Geometry check sheet. Reference: the model listing, model coordinates, mm. Face numbers are marked on the shaded views. A direction names the side the tool comes from. Coordinates: 2 decimals unless noted, no trailing zeros. Loops run counter-clockwise (first coordinate to the right, second up) from the corner with the lowest first, then second, coordinate; pieces in that order, holes last. Notation, with made-up numbers: M 57.5,83 L 110.5,83 A28 cw 110.5,115 Z; hole C 35.5,20.5 d4. An arc over 180 degrees is marked long. Use CSV: the item, a comma, the result in double quotes.
```python
from build123d import *

# Parameters (mm, degrees)
SKETCH1_W           = 16
SKETCH1_H           = 30
BOSS_EXTRUDE1_DEPTH = 9
SKETCH2_R           = 3
BOSS_EXTRUDE2_DEPTH = 1
SKETCH3_R           = 3
BOSS_EXTRUDE3_DEPTH = 2
BOSS_EXTRUDE4_DEPTH = 30
SKETCH6_R           = 0.75
BOSS_EXTRUDE5_DEPTH = 10
SKETCH7_R           = 3.5
BOSS_EXTRUDE6_DEPTH = 4


with BuildPart() as part:
    # Sketch1 → Boss-Extrude1 (new body, symmetric)
    with BuildSketch(Plane(origin=(0, 0, 0), x_dir=(1, 0, 0), z_dir=(0, 1, 0))):
        with Locations((0, -15)):
            Rectangle(SKETCH1_W, SKETCH1_H)
    extrude(amount=BOSS_EXTRUDE1_DEPTH, both=True)

    # Sketch2 → Boss-Extrude2 (add)
    with BuildSketch(Plane(origin=(0, 0, 0), x_dir=(-1, 0, 0), z_dir=(0, 0, -1))):
        Circle(SKETCH2_R)
    extrude(amount=BOSS_EXTRUDE2_DEPTH)

    # Sketch3 → Boss-Extrude3 (add)
    with BuildSketch(Plane.XY.offset(30)):
        Circle(SKETCH3_R)
    extrude(amount=BOSS_EXTRUDE3_DEPTH)

    # Sketch5 → Boss-Extrude4 (add)
    with BuildSketch(Plane.XY):
        with BuildLine():
            Line((8, 9), (8, -9))
            ThreePointArc((8, -9), (12, 0), (8, 9))
        make_face()
        with BuildLine():
            Line((-8, 9), (-8, -9))
            ThreePointArc((-8, -9), (-12, 0), (-8, 9))
        make_face()
    extrude(amount=BOSS_EXTRUDE4_DEPTH)

    # Sketch6 → Boss-Extrude5 (add)
    with BuildSketch(Plane(origin=(0, 0, 0), x_dir=(-1, 0, 0), z_dir=(0, 0, -1))):
        Circle(SKETCH6_R)
    extrude(amount=BOSS_EXTRUDE5_DEPTH)

    # Sketch7 → Boss-Extrude6 (add)
    with BuildSketch(Plane(origin=(0, 0, -10), x_dir=(-1, 0, 0), z_dir=(0, 0, -1))):
        Circle(SKETCH7_R)
    extrude(amount=-BOSS_EXTRUDE6_DEPTH)


solid = part.part
```
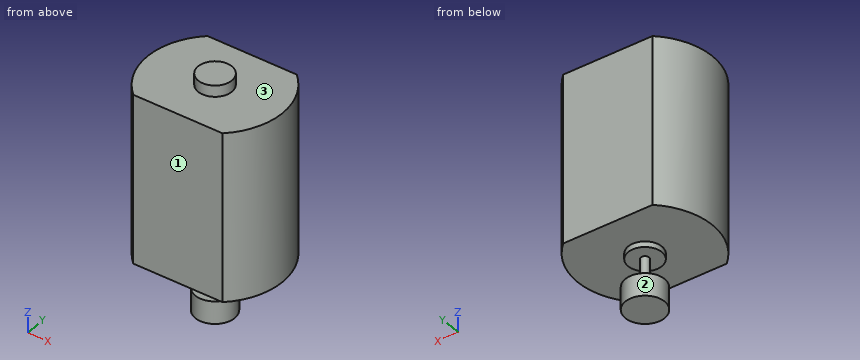
1. Set-up check for the marked faces 1, 2 and 3: record each of +Z, -Z, +X, -X, +Y, -Y from which the full face is reachable in a straight line by a thin tool's end or side.
The answers:
face 1,"+Z, -Z, +X, -X, -Y"
face 2,"-Z"
face 3,"+Z"
2. Thickness scan on line 1 (Z direction, x = 0.25, y = 1); line 2 (Z direction, x = 2.75, y = 2); line 3 (Z direction, x = 0.5, y = 7.25). Record the ranges inside material, lowest first. Write a range as [from, to].
The answers:
line 1,"[-10, -6], [-1, 32]"
line 2,"[-10, -6], [0, 30]"
line 3,"[0, 30]"
3. Section check B-B, the plane x = 0. Record the cut outline in (y, z), plus the area to 4 significant figures.
The answers:
outline,"M -9,0 L -3,0 L -3,-1 L -0.75,-1 L -0.75,-6 L -3.5,-6 L -3.5,-10 L 3.5,-10 L 3.5,-6 L 0.75,-6 L 0.75,-1 L 3,-1 L 3,0 L 9,0 L 9,30 L 3,30 L 3,32 L -3,32 L -3,30 L -9,30 Z"
area,"593.5 mm^2"
4. Section check D-D, the plane x = 5.75. Record the cut outline in (y, z), plus the area to 3 significant figures.
The answers:
outline,"M -9,0 L 9,0 L 9,30 L -9,30 Z"
area,"540 mm^2"
5. Gauge pin test, flat end, axial feed: P1, Ø6, axis at y = -3.5, z = -5, coming from the -X side. Record the tip position at first contact, or that the pin passes through.
The answers:
P1,"x = -3.43"
6. Section check C-C, the plane z = 5.5. Record the cut outline in (x, y) (3 decimals).
The answers:
outline,"M -8,-9 L 8,-9 A12.125 ccw 8,9 L -8,9 A12.125 ccw Z"
7. Section check A-A, the plane y = 0. Record the cut outline in (x, z).
The answers:
outline,"M -12,0 L -3,0 L -3,-1 L -0.75,-1 L -0.75,-6 L -3.5,-6 L -3.5,-10 L 3.5,-10 L 3.5,-6 L 0.75,-6 L 0.75,-1 L 3,-1 L 3,0 L 12,0 L 12,30 L 3,30 L 3,32 L -3,32 L -3,30 L -12,30 Z"
